Check sheet for the modelled part. Datum: model origin and axes. Units: mm. A direction names the side the tool comes from. Give positions to 0.01 mm unless a question says otherwise; leave off trailing zeros. Order: outer loops, then holes, each group sorted by start corner. A loop starts at its lowest first (then second) coordinate and runs counter-clockwise, first axis right, second up. Notation, with made-up numbers: M 67.5,5.25 L 108.5,5.25 A37 ccw 108.5,42.25 Z; hole C 89.5,-34.75 d8. An arc over 180 degrees is marked long. Answer in a Markdown table with one row per item. Add a question column.
Autodesk Inventor part; units mm, degrees
ref_plane "YZ Plane" through (0, 0, 0) normal (1, 0, 0) x (0, 1, 0)
ref_plane "XZ Plane" through (0, 0, 0) normal (0, 1, 0) x (-1, 0, 0)
ref_plane "XY Plane" through (0, 0, 0) normal (0, 0, 1) x (1, 0, 0)
sketch "スケッチ1" plane through (0, 0, 0) normal (0, 0, 1) x (1, 0, 0)
  line L0 (0, 0) -> (300, 0)
  line L1 (300, 0) -> (300, 175)
  line L2 (300, 175) -> (0, 175)
  line L3 (0, 175) -> (0, 0)
  dimension "d0" = 175
  dimension "d1" = 300
extrude "押し出し1" add sketch "スケッチ1" along normal blind 5
sketch "スケッチ2" plane through (0, 0, 5) normal (0, 0, 1) x (1, 0, 0)
  line L0 (-6.3861, 0) -> (323.6139, 0)
  circle A0 centre (75, 60) radius 46
  circle A1 centre (225, 60) radius 46
  line L1 (75, 60) -> (75, 156.1238)
  line L2 (225, 60) -> (225, 147.3766)
  line L3 (75, 60) -> (50.2691, 119.7057)
  line L4 (225, 60) -> (203.3576, 112.2494)
  circle A2 centre (57.3966, 102.4985) radius 1.6
  circle A3 centre (207.3966, 102.4985) radius 1.6
  circle A4 centre (32.5015, 77.6034) radius 1.6
  circle A5 centre (32.5015, 42.3966) radius 1.6
  circle A6 centre (57.3966, 17.5015) radius 1.6
  circle A7 centre (92.6034, 17.5015) radius 1.6
  circle A8 centre (117.4985, 42.3966) radius 1.6
  circle A9 centre (117.4985, 77.6034) radius 1.6
  circle A10 centre (92.6034, 102.4985) radius 1.6
  circle A11 centre (182.5015, 77.6034) radius 1.6
  circle A12 centre (182.5015, 42.3966) radius 1.6
  circle A13 centre (207.3966, 17.5015) radius 1.6
  circle A14 centre (242.6034, 17.5015) radius 1.6
  circle A15 centre (267.4985, 42.3966) radius 1.6
  circle A16 centre (267.4985, 77.6034) radius 1.6
  circle A17 centre (242.6034, 102.4985) radius 1.6
  circle A18 centre (75, 60) radius 30
  circle A19 centre (225, 60) radius 30
  line L5 (323.6139, 175) -> (-6.3861, 175)
  line L6 (-6.3861, 145) -> (19.1813, 0)
  line L7 (323.6139, 145) -> (298.0465, 0)
  line L8 (0, 175) -> (0, 0)
  line L9 (300, 175) -> (300, 0)
  line L10 (300, 175) -> (0, 175)
  line L11 (0, 175) -> (0, 0)
  dimension "d10" = 92
  dimension "d11" = 92
  dimension "d8" = 60
  dimension "d9" = 60
  dimension "d12" = 22.5
  dimension "d13" = 22.5
  dimension "d14" = 3.2
  dimension "d15" = 3.2
  dimension "d16" = 360
  dimension "d17" = 360
  dimension "d18" = 60
  dimension "d19" = 60
  dimension "d20" = 175
  dimension "d21" = 30
  dimension "d22" = 30
  dimension "d23" = 80
  dimension "d24" = 80
  dimension "d25" = 300
  dimension "d26" = 0
  dimension "d27" = 0
  dimension "d28" = 150
  dimension "d29" = 75
extrude "押し出し2" cut sketch "スケッチ2" against normal blind 5 contours A9 A0 | A0 A9 | A8 A0 | A0 A8 | A7 A0 | A0 A7 | A6 A0 | A0 A6 | A18 L3 L1 | L1 L3 A18 | A5 A0 | A0 A5 | A4 A0 | A0 A4 | A16 A1 | A1 A16 | A15 A1 | A1 A15 | A14 A1 | A1 A14 | A13 A1 | A1 A13 | A19 L4 L2 | L2 L4 A19 | A12 A1 | A1 A12 | A11 A1 | A1 A11
sketch "スケッチ3" plane through (0, 0, 5) normal (0, 0, 1) x (1, 0, 0)
  circle A0 centre (75, 60) radius 30
  line L0 (75, 60) -> (100, 60)
  line L1 (100, 60) -> (100, 110)
  line L2 (100, 110) -> (75, 110)
  line L3 (75, 110) -> (75, 60)
  line L4 (75, 110) -> (50, 110)
  line L5 (50, 110) -> (50, 60)
  line L6 (50, 60) -> (75, 60)
  line L7 (75, 60) -> (75, 110)
  line L8 (50, 110) -> (42.3811, 36.1629)
  line L9 (100, 110) -> (107.6189, 36.1629)
  line L10 (300, 175) -> (0, 175)
  line L11 (150, 175) -> (150, 0)
  line L12 (0, 0) -> (300, 0)
  line L13 (200, 110) -> (225, 110)
  line L14 (225, 110) -> (250, 110)
  line L15 (250, 110) -> (257.6189, 36.1629)
  line L16 (200, 110) -> (192.3811, 36.1629)
  circle A1 centre (225, 60) radius 30
  circle A2 centre (225, 60) radius 30
  point P0 (45.1584, 63.0792)
  point P1 (104.8416, 63.0792)
  point P2 (195.1584, 63.0792)
  point P3 (254.8416, 63.0792)
  dimension "d32" = 25
  dimension "d33" = 50
  dimension "d34" = 25
extrude "押し出し3" cut sketch "スケッチ3" against normal blind 5 contours A0 L1 L9 | L8 L5 A0 | A0 L3 L2 L1 | L5 L4 L3 A0 | L13 L14 L15 A1 L16
sketch "スケッチ4" plane through (0, 0, 5) normal (0, 0, 1) x (1, 0, 0)
  line L0 (0, 175) -> (0, 0)
  line L1 (300, 0) -> (300, 175)
  line L2 (0, 175) -> (300, 175)
  line L3 (300, 175) -> (300, 110)
  line L4 (300, 110) -> (0, 110)
  line L5 (0, 110) -> (0, 175)
  line L6 (0, 135) -> (300, 135)
  line L7 (300, 135) -> (300, 115)
  line L8 (300, 115) -> (0, 115)
  line L9 (0, 115) -> (0, 135)
  line L10 (40, 135) -> (110, 135)
  line L11 (110, 135) -> (110, 115)
  line L12 (110, 115) -> (40, 115)
  line L13 (40, 115) -> (40, 135)
  line L14 (150, 115) -> (150, 0)
  line L15 (190, 135) -> (190, 115)
  line L16 (260, 115) -> (260, 135)
  dimension "d38" = 65
  dimension "d39" = 20
  dimension "d40" = 5
  dimension "d41" = 70
  dimension "d192" = 40
extrude "押し出し4" cut sketch "スケッチ4" against normal blind 5 contours L6 L11 L8 L13 | L16 L8 L15 L6
fillet "フィレット2" radius 5 12 edges at (110, 135, 2.5) (260, 135, 2.5) (260, 115, 2.5) (190, 135, 2.5) (190, 115, 2.5) (40, 115, 2.5) (40, 135, 2.5) (110, 115, 2.5) (100, 110, 2.5) (250, 110, 2.5) (200, 110, 2.5) (50, 110, 2.5)
sketch "スケッチ5" plane through (0, 0, 5) normal (0, 0, 1) x (1, 0, 0)
  line L0 (300, 175) -> (0, 175)
  line L1 (300, 0) -> (300, 175)
  line L2 (0, 175) -> (300, 175)
  line L3 (300, 175) -> (300, 170)
  line L4 (300, 170) -> (0, 170)
  line L5 (0, 170) -> (0, 175)
  line L6 (20, 175) -> (20, 170)
  line L7 (40, 175) -> (40, 170)
  line L8 (60, 175) -> (60, 170)
  line L9 (80, 175) -> (80, 170)
  line L10 (100, 175) -> (100, 170)
  line L11 (120, 175) -> (120, 170)
  line L12 (140, 175) -> (140, 170)
  line L13 (160, 175) -> (160, 170)
  line L14 (180, 175) -> (180, 170)
  line L15 (200, 175) -> (200, 170)
  line L16 (220, 175) -> (220, 170)
  line L17 (240, 175) -> (240, 170)
  line L18 (260, 175) -> (260, 170)
  line L19 (280, 175) -> (280, 170)
  line L20 (300, 175) -> (300, 170)
  point P0 (0, 0)
  point P1 (0, 172.5)
  dimension "d46" = 5
  dimension "d47" = 20
  dimension "d50" = 20
extrude "押し出し5" cut sketch "スケッチ5" against normal blind 5
fillet "フィレット6" radius 10 2 edges at (0, 0, 2.5) (300, 0, 2.5)
fillet "フィレット7" radius 2 2 edges at (300, 170, 2.5) (0, 170, 2.5)
equation "\"d11\" = d10"
equation "\"d8\" = d9"
equation "\"d15\" = d14"
equation "\"d24\" = d23"
equation "\"d34\" = d32"
properties part number "RP_Waist-Under" material "A5052"
Q1. Draft check along Y on faces 3 (the cylindrical face through (296.99, 2.85, 2.54)), 4 (the flat face through (148, 86, 0)), 5 (the cylindrical face through (74.3, 30.01, 2.54)). Enter one of: pulls with the +Y half, pulls with the -Y half, needs draft (parallel to the pull), parting line crosses it, or undercut.
Q2. Thickness scan on probe 1 along X at (y, z) = (105.5, 0.6); probe 2 along Y at (x, z) = (75, 2); probe 3 along X at (y, z) = (60, 3.25). Record the ranges inside material, lowest first.
Q3. Cross-section at C-C (z = 0.8). State how many separate pieces and enclosed holes the cut face has, and give its area (3 significant figures).
Q4. Cross-section at A-A (y = 60). Record the boundary of the cut face in (x, z), and give its area (3 significant figures).
Q5. Go/stop test with a flat-tipped pin: pin 1 (1.9 mm diameter, centred on x = 117.5, y = 42.4, fed in from -Z). Record where the tip stops, or that it passes through.
Q6. Tool access check on faces 1 (the flat face through (148, 86, 5)), 2 (the cylindrical face through (224.3, 30.01, 2.54)). Record the directions out of +Z, -Z, +X, -X, +Y, -Y that give a thin tool (end or side, any length) a straight path to the whole face; none if there is none.
Q7. Cross-section at B-B (x = 75). Record the boundary of the cut face in (y, z), and give its area (3 significant figures).
Values follow:
| question | item | result |
|---|---|---|
| 1 | face 3 | pulls with the -Y half |
| 1 | face 4 | needs draft |
| 1 | face 5 | undercut |
| 2 | probe 1 | 0 to 49.54, 100.46 to 199.54, 250.46 to 300 |
| 2 | probe 2 | 0 to 30, 110 to 115, 135 to 170 |
| 2 | probe 3 | 0 to 45, 105 to 195, 255 to 300 |
| 3 | separate pieces | 1 |
| 3 | enclosed holes | 16 |
| 3 | area | 39,800 mm² |
| 4 | outline | M 0,0 L 45,0 L 45,5 L 0,5 Z; M 105,0 L 195,0 L 195,5 L 105,5 Z; M 255,0 L 300,0 L 300,5 L 255,5 Z |
| 4 | area | 900 mm² |
| 5 | pin 1 | through |
| 6 | face 1 | +Z, +X, -X, +Y, -Y |
| 6 | face 2 | +Z, -Z |
| 7 | outline | M 0,0 L 30,0 L 30,5 L 0,5 Z; M 110,0 L 115,0 L 115,5 L 110,5 Z; M 135,0 L 170,0 L 170,5 L 135,5 Z |
| 7 | area | 350 mm² |
